Geometry check sheet. Reference: the model listing, model coordinates, mm. A direction names the side the tool comes from. Round coordinates to 2 decimals unless told otherwise and drop trailing zeros. Order: outer loops, then holes, each group sorted by start corner. A loop starts at its lowest first (then second) coordinate and runs counter-clockwise, first axis right, second up. Notation, with made-up numbers: (-5, 57.25) -> (48, 57.25) arc R19 cw to (48, 64.25) -> close; hole circle Ø6 at (30, 61.5). An arc over 180 degrees is marked (long way). Use a Markdown table: item, result. Add a question column.
Item 1: Gauge pin test, flat ends, axial feed: pin 1 Ø1 at (x, y) = (4.5, 3.5) entering from -Z; pin 2 Ø1 at (x, y) = (-3.5, 4) entering from -Z; pin 3 Ø1.5 at (x, z) = (-1, -5) entering from -Y. Record the tip position at first contact, or that the pin passes through.
Item 2: Sectioned sample at A-A, the plane z = 0. Record the cut outline in (x, y), and give its area (3 significant figures).
Item 3: Set-up check for faces 1 (the flat face through (1, 0, 3)), 2 (the flat face through (3, 0.25, 3)): record each of +Z, -Z, +X, -X, +Y, -Y from which the full face is reachable in a straight line by a thin tool's end or side.
Item 4: Sectioned sample at C-C, the plane y = 0.9. Record the cut outline in (x, z), and give its area (3 significant figures).
Item 5: Material ranges on probe 1 along Z at (x, y) = (-2.75, 4.8); probe 2 along X at (y, z) = (3.15, 0); probe 3 along Y at (x, z) = (-4.75, 2.5), recorded low to high. Write a range as [from, to].
Item 6: Sectioned sample at D-D, the plane z = 4. Record the cut outline in (x, y).
Item 7: Mould release check, pull along X, two halves, no side actions. Record for faces 3 (the flat face through (-6, 5, 2)), 4 (the flat face through (3, 4.75, 3)), 5 (the cylindrical face through (-3.955, 2.465, -5.158)): pulls with the +X half, pulls with the -X half, needs draft (parallel to the pull), parting line crosses it, or undercut.
Item 8: Sectioned sample at B-B, the plane x = 0. Record the cut outline in (y, z), and give its area (3 significant figures).
from build123d import *

# Parameters (mm, degrees)
SKETCH1_R           = 6.5
SKETCH1_R_2         = 3
BOSS_EXTRUDE1_DEPTH = 5
SKETCH2_W           = 2.5
SKETCH2_H           = 0.25


with BuildPart() as part:
    # Sketch1 → Boss-Extrude1 (new body)
    with BuildSketch(Plane(origin=(0, 0, 0), x_dir=(1, 0, 0), z_dir=(0, 1, 0))):
        with Locations(Location((0, 0, 0), (0, 0, 270))):
            Circle(SKETCH1_R)
        with Locations(Location((0, 0, 0), (0, 0, 270))):
            Circle(SKETCH1_R_2, mode=Mode.SUBTRACT)
    extrude(amount=BOSS_EXTRUDE1_DEPTH)

    # Sketch2 → Cut-Revolve1 (revolve, cut)
    with BuildSketch(Plane.XY, mode=Mode.PRIVATE) as cut_revolve1_sk:
        with Locations((-4.75, 4.875)):
            Rectangle(SKETCH2_W, SKETCH2_H)
        with Locations((-4.75, 0.125)):
            Rectangle(SKETCH2_W, SKETCH2_H)
    revolve(cut_revolve1_sk.sketch.rotate(Axis((0, 5, 0), (0, -1, 0)), 270), axis=Axis((0, 5, 0), (0, -1, 0)), mode=Mode.SUBTRACT)


solid = part.part
Found:
| question | item | result |
|---|---|---|
| 1 | pin 1 | stops at z = -5.12 |
| 1 | pin 2 | stops at z = -5.77 |
| 1 | pin 3 | stops at y = 0.25 |
| 2 | outline | (-6.5, 0) -> (-6, 0) -> (-6, 0.25) -> (-3.5, 0.25) -> (-3.5, 0) -> (-3, 0) -> (-3, 5) -> (-3.5, 5) -> (-3.5, 4.75) -> (-6, 4.75) -> (-6, 5) -> (-6.5, 5) -> close; (3, 0) -> (3.5, 0) -> (3.5, 0.25) -> (6, 0.25) -> (6, 0) -> (6.5, 0) -> (6.5, 5) -> (6, 5) -> (6, 4.75) -> (3.5, 4.75) -> (3.5, 5) -> (3, 5) -> close |
| 2 | area | 32.5 mm2 |
| 3 | face 1 | +Z, -Z, +X, -X, -Y |
| 3 | face 2 | -Y |
| 4 | outline | circle Ø13 at (0, 0); hole circle Ø6 at (0, 0) |
| 4 | area | 104 mm2 |
| 5 | probe 1 | z = [-5.89, -5.33], [-2.17, -1.2], [1.2, 2.17], [5.33, 5.89] |
| 5 | probe 2 | x = [-6.5, -3], [3, 6.5] |
| 5 | probe 3 | y = [0.25, 4.75] |
| 6 | outline | (-5.12, 0) -> (-4.47, 0) -> (-4.47, 0.25) -> (4.47, 0.25) -> (4.47, 0) -> (5.12, 0) -> (5.12, 5) -> (4.47, 5) -> (4.47, 4.75) -> (-4.47, 4.75) -> (-4.47, 5) -> (-5.12, 5) -> close |
| 7 | face 3 | needs draft |
| 7 | face 4 | undercut |
| 7 | face 5 | parting line crosses it |
| 8 | outline | (0, -6.5) -> (5, -6.5) -> (5, -6) -> (4.75, -6) -> (4.75, -3.5) -> (5, -3.5) -> (5, -3) -> (0, -3) -> (0, -3.5) -> (0.25, -3.5) -> (0.25, -6) -> (0, -6) -> close; (0, 3) -> (5, 3) -> (5, 3.5) -> (4.75, 3.5) -> (4.75, 6) -> (5, 6) -> (5, 6.5) -> (0, 6.5) -> (0, 6) -> (0.25, 6) -> (0.25, 3.5) -> (0, 3.5) -> close |
| 8 | area | 32.5 mm2 |
